Part model, mm, in its own coordinate system. Coordinates: 2 decimals unless noted, no trailing zeros. Loops run counter-clockwise (first coordinate to the right, second up) from the corner with the lowest first, then second, coordinate; pieces in that order, holes last. Notation, with made-up numbers: M 35,68.5 L 41,68.5 A13 ccw 41,90.5 Z; hole C 79.5,36.5 d9. An arc over 180 degrees is marked long. Use a Markdown table: item, result. Add a question column.
1) Band-saw the part on A-A (x = 0). List the corners of the cut face in (y, z), plus the area to 3 significant figures.
2) Band-saw the part on D-D (z = -9.5). List the corners of the cut face in (x, y).
3) Wall check: probe 1 along Z at (x, y) = (-29.5, 2); probe 2 along X at (y, z) = (0.7, 0); probe 3 along Z at (x, y) = (-31.5, 0.45). Give the ranges that are in metal, low to high. Write a range as from..to.
4) Band-saw the part on C-C (y = 1.2). State how many separate pieces and enclosed holes the cut face has, plus the area to 3 significant figures.
5) Band-saw the part on B-B (z = 0). List the corners of the cut face in (x, y).
from build123d import *

# Parameters (mm, degrees)
BOSS_EXTRUDE1_DEPTH = 2.54
SKETCH2_R           = 3.571875
SKETCH2_R_2         = 3.175
CUT_EXTRUDE4_DEPTH  = 67.782319344


with BuildPart() as part:
    # Sketch1 → Boss-Extrude1 (new body)
    with BuildSketch(Plane(origin=(0, 0, 0), x_dir=(1, 0, 0), z_dir=(0, 1, 0))):
        Polygon((54.991, -19.304), (60.833, -13.462), (60.833, -5.82667054), (54.102, 19.293763446), (-57.15, 19.293763446), (-63.881, -5.82667054), (-63.881, -13.462), (-58.039, -19.304), align=None)
    extrude(amount=BOSS_EXTRUDE1_DEPTH)

    # Sketch2 → Cut-Extrude4 (cut, through all)
    with BuildSketch(Plane(origin=(0, 2.54, 0), x_dir=(1, 0, 0), z_dir=(0, 1, 0))):
        with Locations(Location((-29.1465, -0.005118277, 0), (0, 0, 270))):
            Circle(SKETCH2_R)
        with Locations(Location((0, 0, 0), (0, 0, 270))):
            Circle(SKETCH2_R)
        with Locations(Location((26.7335, -0.005118277, 0), (0, 0, 270))):
            Circle(SKETCH2_R_2)
    extrude(amount=-CUT_EXTRUDE4_DEPTH, mode=Mode.SUBTRACT)


solid = part.part
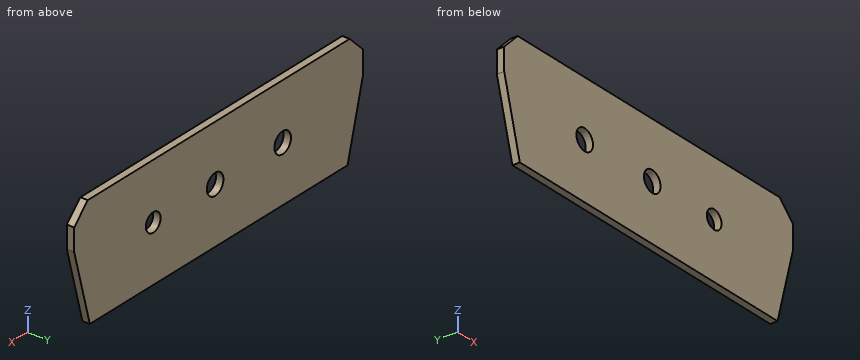
Entries:
| question | item | result |
|---|---|---|
| 1 | outline | M 0,-19.29 L 2.54,-19.29 L 2.54,-3.57 L 0,-3.57 Z; M 0,3.57 L 2.54,3.57 L 2.54,19.3 L 0,19.3 Z |
| 1 | area | 79.9 mm2 |
| 2 | outline | M -59.77,0 L 56.73,0 L 56.73,2.54 L -59.77,2.54 Z |
| 3 | probe 1 | -19.29..-3.55, 3.56..19.3 |
| 3 | probe 2 | -62.32..-32.72, -25.57..-3.57, 3.57..23.56, 29.91..59.27 |
| 3 | probe 3 | -19.29..-2.68, 2.69..19.3 |
| 4 | separate pieces | 1 |
| 4 | enclosed holes | 3 |
| 4 | area | 4,500 mm2 |
| 5 | outline | M -62.32,0 L -32.72,0 L -32.72,2.54 L -62.32,2.54 Z; M -25.57,0 L -3.57,0 L -3.57,2.54 L -25.57,2.54 Z; M 3.57,0 L 23.56,0 L 23.56,2.54 L 3.57,2.54 Z; M 29.91,0 L 59.27,0 L 59.27,2.54 L 29.91,2.54 Z |
